```python
from build123d import *

# Parameters (mm, degrees)
SKETCH1_W           = 126.56
SKETCH1_H           = 85
BOSS_EXTRUDE1_DEPTH = 3
SKETCH2_W           = 123.16
SKETCH2_H           = 81.6
BOSS_EXTRUDE2_DEPTH = 8.45
CUT_EXTRUDE1_DEPTH  = 8.45
FILLET1_R           = 1
SHELL1_T            = -2
FILLET2_R           = 2
SKETCH4_W           = 24.75
SKETCH4_H           = 60.75
CUT_EXTRUDE2_DEPTH  = 1
SKETCH5_W           = 22.75
SKETCH5_H           = 58.75
CUT_EXTRUDE3_DEPTH  = 1
BOSS_EXTRUDE4_DEPTH = 5


with BuildPart() as part:
    # Sketch1 → Boss-Extrude1 (new body)
    with BuildSketch(Plane.XY):
        with Locations((63.28, 42.5)):
            Rectangle(SKETCH1_W, SKETCH1_H)
    extrude(amount=BOSS_EXTRUDE1_DEPTH)

    # Sketch2 → Boss-Extrude2 (add)
    with BuildSketch(Plane.XY.offset(3)):
        with Locations((63.28, 42.5)):
            Rectangle(SKETCH2_W, SKETCH2_H)
    extrude(amount=BOSS_EXTRUDE2_DEPTH)

    # Sketch3 → Cut-Extrude1 (cut)
    with BuildSketch(Plane.XY.offset(11.45)):
        Polygon((1.7, 83.3), (1.7, 74.8), (10.2, 83.3), align=None)
        Polygon((124.86, 83.3), (116.36, 83.3), (124.86, 74.8), align=None)
        Polygon((124.86, 1.7), (124.86, 10.2), (116.36, 1.7), align=None)
    extrude(amount=-CUT_EXTRUDE1_DEPTH, mode=Mode.SUBTRACT)

    # Fillet1
    fillet1_edges = [part.edges().sort_by_distance(p)[0] for p in [
        (1.7, 1.7, 7.225),
        (10.2, 83.3, 7.225),
        (1.7, 74.8, 7.225),
        (124.86, 74.8, 7.225),
        (116.36, 83.3, 7.225),
        (116.36, 1.7, 7.225),
        (124.86, 10.2, 7.225),
    ]]
    fillet(fillet1_edges, radius=FILLET1_R)

    # Shell1
    shell1_openings = [part.faces().sort_by_distance(p)[0] for p in [
        (63.067597632, 42.362751228, 11.45),
    ]]
    offset(amount=SHELL1_T, openings=shell1_openings, kind=Kind.INTERSECTION)

    # Fillet2
    fillet2_edges = [part.edges().sort_by_distance(p)[0] for p in [
        (0, 85, 1.5),
        (126.56, 85, 1.5),
        (126.56, 0, 1.5),
        (0, 0, 1.5),
    ]]
    fillet(fillet2_edges, radius=FILLET2_R)

    # Sketch4 → Cut-Extrude2 (cut)
    with BuildSketch(Plane.XY.offset(2)):
        with Locations((17.875, 41.925)):
            Rectangle(SKETCH4_W, SKETCH4_H)
        with Locations((47.875, 41.925)):
            Rectangle(SKETCH4_W, SKETCH4_H)
        with Locations((77.875, 41.925)):
            Rectangle(SKETCH4_W, SKETCH4_H)
        with Locations((107.875, 41.925)):
            Rectangle(SKETCH4_W, SKETCH4_H)
    extrude(amount=-CUT_EXTRUDE2_DEPTH, mode=Mode.SUBTRACT)

    # Sketch5 → Cut-Extrude3 (cut)
    with BuildSketch(Plane.XY.offset(1)):
        with Locations((17.875, 41.925)):
            Rectangle(SKETCH5_W, SKETCH5_H)
        with Locations((47.875, 41.925)):
            Rectangle(SKETCH5_W, SKETCH5_H)
        with Locations((77.875, 41.925)):
            Rectangle(SKETCH5_W, SKETCH5_H)
        with Locations((107.875, 41.925)):
            Rectangle(SKETCH5_W, SKETCH5_H)
    extrude(amount=-CUT_EXTRUDE3_DEPTH, mode=Mode.SUBTRACT)

    # Sketch7 → Boss-Extrude4 (add)
    with BuildSketch(Plane.XY.offset(2)):
        Polygon((3.7, 73.971572875), (122.86, 73.971572875), (120.655411021, 76.176161854), (5.904588979, 76.176161854), align=None)
        Polygon((3.7, 9.782267604), (3.7, 7.282267604), (119.195786438, 7.364213562), (121.613840479, 9.782267604), align=None)
    extrude(amount=BOSS_EXTRUDE4_DEPTH)


solid = part.part
```
Design review of the part built by this model. Coordinates are the model's own, in mm. A direction names the side the tool comes from. Round coordinates to 2 decimals unless told otherwise and drop trailing zeros. Order: outer loops, then holes, each group sorted by start corner. A loop starts at its lowest first (then second) coordinate and runs counter-clockwise, first axis right, second up. Notation, with made-up numbers: (6.5, 57) - (47.5, 57) arc R11 ccw to (47.5, 71) - close; hole circle Ø2 at (60.5, -1). An arc over 180 degrees is marked (long way). Return JSON: item names as keys, results as strings.
Q1. Consider section B-B on z = 4.25. Write out the cut boundary in (x, y).
Computed values:
{"outline": "(1.7, 2.7) arc R1 ccw to (2.7, 1.7) - (115.95, 1.7) arc R1 ccw to (116.65, 1.99) - (124.57, 9.91) arc R1 ccw to (124.86, 10.61) - (124.86, 74.39) arc R1 ccw to (124.57, 75.09) - (116.65, 83.01) arc R1 ccw to (115.95, 83.3) - (10.61, 83.3) arc R1 ccw to (9.91, 83.01) - (1.99, 75.09) arc R1 ccw to (1.7, 74.39) - close; hole (3.7, 3.7) - (115.53, 3.7) - (119.2, 7.36) - (3.7, 7.28) - close; hole (3.7, 9.78) - (121.61, 9.78) - (122.86, 11.03) - (122.86, 73.97) - (3.7, 73.97) - close; hole (5.9, 76.18) - (120.66, 76.18) - (115.53, 81.3) - (11.03, 81.3) - close"}
Q2. Consider section D-D on y = 79. Write out the cut boundary in (x, z), plus the area to 3 significant figures.
Computed values:
{"outline": "(0, 0) - (126.56, 0) - (126.56, 3) - (120.66, 3) - (120.66, 11.45) - (117.83, 11.45) - (117.83, 2) - (8.73, 2) - (8.73, 11.45) - (5.9, 11.45) - (5.9, 3) - (0, 3) - close", "area": "318 mm2"}
Q3. Machinability: for faces 4 (the flat face through (120.55, 79.11, 7.28)), 5 (the flat face through (124.86, 42, 7)), 6 (the flat face through (59, 1.7, 7)), 7 (the flat face through (64, 76.176, 4)), which of the approach directions +Z, -Z, +X, -X, +Y, -Y give a long, thin tool a straight path to every point of the face, cutting with its end or side? Answer none if there is none.
Computed values:
{"face 4": "+Z, +X, +Y", "face 5": "+Z, +X, +Y, -Y", "face 6": "+Z, +X, -X, -Y", "face 7": "+Z"}
Q4. Consider section C-C on y = 33.5. Give the number of separate pieces and of enclosed holes in the cut face, plus the area to 3 significant figures.
Computed values:
{"separate pieces": "5", "enclosed holes": "0", "area": "104 mm2"}
Q5. For pin 1 Ø1 at (y, z) = (31, 4.5) entering from +X; pin 2 Ø2.5 at (x, z) = (76.5, 5.5) entering from +Y; pin 3 Ø2 at (x, z) = (99.5, 3.5) entering from -Y; pin 4 Ø5 at (x, z) = (65, 9.5) entering from -Y, all flat-tipped, find the tip position at first contact; note any pin that passes through.
Computed values:
{"pin 1": "stops at x = 124.86", "pin 2": "stops at y = 83.3", "pin 3": "stops at y = 0", "pin 4": "stops at y = 1.7"}
Q6. Consider section A-A on z = 9.75. Write out the cut boundary in (x, y).
Computed values:
{"outline": "(1.7, 2.7) arc R1 ccw to (2.7, 1.7) - (115.95, 1.7) arc R1 ccw to (116.65, 1.99) - (124.57, 9.91) arc R1 ccw to (124.86, 10.61) - (124.86, 74.39) arc R1 ccw to (124.57, 75.09) - (116.65, 83.01) arc R1 ccw to (115.95, 83.3) - (10.61, 83.3) arc R1 ccw to (9.91, 83.01) - (1.99, 75.09) arc R1 ccw to (1.7, 74.39) - close; hole (3.7, 3.7) - (115.53, 3.7) - (122.86, 11.03) - (122.86, 73.97) - (115.53, 81.3) - (11.03, 81.3) - (3.7, 73.97) - close"}
Q7. Wall thickness on L1, parallel to Y at x = 29, z = 5.75; L2, parallel to Y at x = 31, z = 2.25; L3, parallel to Y at x = 106.5, z = 11.25: over which ranges is each line inside the solid? List them lowest first. Write a range as [from, to].
Computed values:
{"L1": "y = [1.7, 3.7], [7.3, 9.78], [73.97, 76.18], [81.3, 83.3]", "L2": "y = [0, 3.7], [7.3, 9.78], [73.97, 76.18], [81.3, 85]", "L3": "y = [1.7, 3.7], [81.3, 83.3]"}
Q8. The part is to be moulded in two halves that separate along X. For faces 1 (the flat face through (1.7, 38, 7)), 2 (the flat face through (120, 51, 1)), 3 (the flat face through (62, 85, 1)), say which applies: pulls with the +X half, pulls with the -X half, needs draft (parallel to the pull), parting line crosses it, or undercut.
Computed values:
{"face 1": "pulls with the -X half", "face 2": "undercut", "face 3": "needs draft"}
